Design review of the part built by this model. Coordinates are the model's own, in mm. Face numbers are marked on the shaded views. A direction names the side the tool comes from. Coordinates: 2 decimals unless noted, no trailing zeros. Loops run counter-clockwise (first coordinate to the right, second up) from the corner with the lowest first, then second, coordinate; pieces in that order, holes last. Notation, with made-up numbers: (15.5, 42) -> (59.5, 42) arc R20 cw to (59.5, 57) -> close; hole circle Ø4 at (42.25, 58.25). An arc over 180 degrees is marked (long way). Use one line per item in the form item = value. Start each with the question number.
1. Machinability: for the marked faces 4 and 5, which of the approach directions +Z, -Z, +X, -X, +Y, -Y give a long, thin tool a straight path to every point of the face, cutting with its end or side? Answer none if there is none.
2. For pin 1 (5 mm diameter, centred on x = 3.5, z = 6.5, fed in from -Y); pin 2 (3 mm diameter, centred on y = -25.5, z = 6.5, fed in from -X); pin 3 (8 mm diameter, centred on x = 14.5, y = -26, fed in from -Z); pin 4 (6 mm diameter, centred on x = 5.5, z = 5.5, fed in from -Y), all flat-tipped, find the tip position at first contact; note any pin that passes through.
3. Consider section A-A (y = -2.5). State the section outline as (x, z) points, then the cut area to 4 significant figures.
4. Consider section B-B (z = 8.75). State how many separate pieces and enclosed holes the cut face has, then the cut area to 3 significant figures.
5. The part is to be moulded in two halves that separate along X. For the marked faces 1, 2 and 3, say which applies: released by +X, released by -X, zero draft, split by the parting line, or undercut.
6. Wall thickness on line 1 (Z direction, x = 6.75, y = -12.5); line 2 (X direction, y = -2.5, z = 7.25); line 3 (X direction, y = -16.5, z = 8.4): over which ranges is each line inside the solid? List them lowest first. Write a range as from..to.
7. Consider section C-C (x = 6). State the section outline as (y, z) points, then the cut area to 3 significant figures.
8. Consider section D-D (y = -15.5). State the section outline as (x, z) points, then the cut area to 3 significant figures.
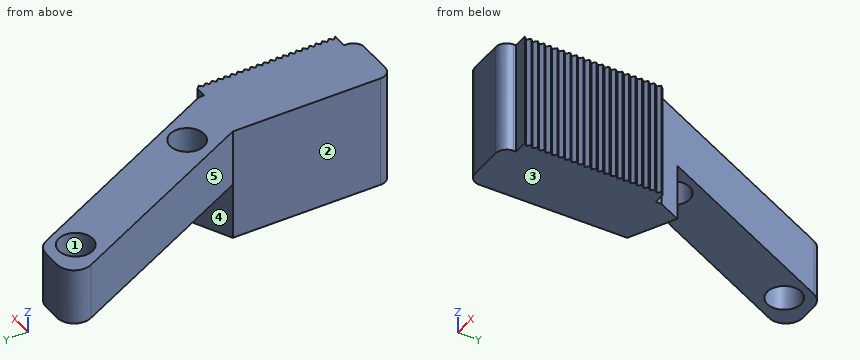
from build123d import *

# Parameters (mm, degrees)
SKETCH2_R           = 1.5
BOSS_EXTRUDE1_DEPTH = 10
SKETCH3_W           = 5
SKETCH3_H           = 22.360679775
CUT_EXTRUDE1_DEPTH  = 10
FILLET2_R           = 1.5
FILLET3_R           = 1
BOSS_EXTRUDE2_DEPTH = 10


with BuildPart() as part:
    # Sketch2 → Boss-Extrude1 (new body)
    with BuildSketch(Plane.XY):
        Polygon((0, 0), (10, -20), (10, -34), (15, -34), (15, -20), (5, 0), align=None)
        with Locations((3.855019194, -2.5)):
            Circle(SKETCH2_R, mode=Mode.SUBTRACT)
        with Locations((10.855019194, -16.5)):
            Circle(SKETCH2_R, mode=Mode.SUBTRACT)
    extrude(amount=BOSS_EXTRUDE1_DEPTH)

    # Sketch3 → Cut-Extrude1 (cut)
    with BuildSketch(Plane(origin=(0, 0, 0), x_dir=(0, 0, 1), z_dir=(-0.894427191, -0.447213595, 0))):
        with Locations((2.5, -11.180339888)):
            Rectangle(SKETCH3_W, SKETCH3_H)
    extrude(amount=-CUT_EXTRUDE1_DEPTH, mode=Mode.SUBTRACT)

    # Fillet2
    fillet2_edges = [part.edges().sort_by_distance(p)[0] for p in [
        (0, 0, 7.5),
        (5, 0, 7.5),
    ]]
    fillet(fillet2_edges, radius=FILLET2_R)

    # Fillet3
    fillet3_edges = [part.edges().sort_by_distance(p)[0] for p in [
        (15, -34, 5),
        (10, -34, 5),
    ]]
    fillet(fillet3_edges, radius=FILLET3_R)

    # Sketch4 → Boss-Extrude2 (add)
    with BuildSketch(Plane.XY.offset(10)):
        Polygon((15, -20.5), (16, -20.5), (16.271607252, -20.771607252), (16, -21.043214505), (16.290943636, -21.334158141), (16.008789905, -21.616311872), (16.295338588, -21.902860555), (16.008789905, -22.189409238), (16.295338588, -22.475957922), (16.008789905, -22.762506605), (16.295338588, -23.049055289), (16.008789905, -23.335603972), (16.295338588, -23.622152655), (16.008789905, -23.908701339), (16.295338588, -24.195250022), (16.008789905, -24.481798706), (16.295338588, -24.768347389), (16.008789905, -25.054896072), (16.295338588, -25.341444756), (16.008789905, -25.627993439), (16.295338588, -25.914542122), (16.008789905, -26.201090806), (16.295338588, -26.487639489), (16.008789905, -26.774188173), (16.295338588, -27.060736856), (16.008789905, -27.347285539), (16.295338588, -27.633834223), (16.008789905, -27.920382906), (16.295338588, -28.20693159), (16.008789905, -28.493480273), (16.295338588, -28.780028956), (16.008789905, -29.06657764), (16.295338588, -29.353126323), (16.008789905, -29.639675006), (16.295338588, -29.92622369), (16.008789905, -30.212772373), (16.295338588, -30.499321057), (16.008789905, -30.78586974), (16.295338588, -31.072418423), (16.008789905, -31.358967107), (16.295338588, -31.64551579), (16.008789905, -31.932064474), (16.295338588, -32.218613157), (16.008789905, -32.50516184), (16.295338588, -32.791710524), (15, -32.791710524), align=None)
    extrude(amount=-BOSS_EXTRUDE2_DEPTH)


solid = part.part
Geometry check:
q1.face_4 = -Z, -X, +Y
q1.face_5 = +Z, -Z, -X, -Y
q2.pin_1 = -12
q2.pin_2 = 10
q2.pin_3 = 0
q2.pin_4 = -17
q3.outline = (1.25, 5) -> (2.36, 5) -> (2.36, 10) -> (1.25, 10) -> close; (5.36, 5) -> (6.25, 5) -> (6.25, 10) -> (5.36, 10) -> close
q3.area = 10.00 mm²
q4.separate_pieces = 1
q4.enclosed_holes = 2
q4.area = 168 mm²
q5.face_1 = undercut
q5.face_2 = released by -X
q5.face_3 = zero draft
q6.line_1 = 5..10
q6.line_2 = 1.25..2.36, 5.36..6.25
q6.line_3 = 8.25..9.36, 12.36..13.25
q7.outline = (-12, 5) -> (-2, 5) -> (-2, 10) -> (-12, 10) -> close
q7.area = 50.0 mm²
q8.outline = (7.75, 5) -> (9.74, 5) -> (9.74, 10) -> (7.75, 10) -> close; (11.97, 5) -> (12.75, 5) -> (12.75, 10) -> (11.97, 10) -> close
q8.area = 13.8 mm²
